Geometry check sheet. Reference: the model listing, model coordinates, mm. A direction names the side the tool comes from. Coordinates: 2 decimals unless noted, no trailing zeros. Write each loop counter-clockwise with the first axis right and the second up, starting at its lowest first coordinate (ties: lowest second). Pieces come first, ordered by that corner, then holes. Notation, with made-up numbers: M -38.5,34.5 L -14.5,34.5 A28 ccw -14.5,53.5 Z; hole C 76.25,80 d3. An arc over 180 degrees is marked long. Answer as a JSON object with one key per item and string values. Group by question number.
Autodesk Fusion 360 part; units mm, degrees
sketch "Sketch1" plane through (0, 0, 0) normal (0, 0, 1) x (1, 0, 0)
  line L0 (0, 0) -> (-70, 0)
  line L1 (-70, 0) -> (-70, 45)
  line L2 (-70, 45) -> (0, 45)
  line L3 (0, 45) -> (0, 0)
extrude "Extrude1" add sketch "Sketch1" along normal blind 75
sketch "Sketch2" plane through (0, 0, 75) normal (0, 0, 1) x (-1, 0, 0)
  line L0 (0, -45) -> (70, -45)
  line L1 (70, -45) -> (70, 0)
  line L2 (70, 0) -> (0, 0)
  line L3 (0, 0) -> (0, -45)
  line L4 (68, -43) -> (2, -43)
  line L5 (2, -43) -> (2, -2)
  line L6 (2, -2) -> (68, -2)
  line L7 (68, -2) -> (68, -43)
extrude "Extrude2" cut sketch "Sketch2" against normal blind 74.8 contours L4 L5 L6 L7
sketch "Sketch3" plane through (0, 0, 0.2) normal (0, 0, 1) x (-1, 0, 0)
  line L0 (68, -2) -> (2, -2)
  line L1 (2, -2) -> (2, -43)
  line L2 (2, -43) -> (68, -43)
  line L3 (68, -43) -> (68, -2)
  line L4 (68, -21) -> (65, -21)
  line L5 (65, -21) -> (65, -20)
  line L6 (65, -20) -> (68, -20)
  line L7 (68, -20) -> (68, -21)
  line L8 (67, -21) -> (68, -21)
  line L9 (68, -21) -> (68, -22)
  line L10 (68, -22) -> (67, -22)
  line L11 (67, -22) -> (67, -21)
  line L12 (68, -23) -> (65, -23)
  line L13 (65, -23) -> (65, -22)
  line L14 (65, -22) -> (68, -22)
  line L15 (68, -22) -> (68, -23)
  line L16 (19, -22) -> (16, -22)
  line L17 (16, -22) -> (16, -23)
  line L18 (16, -23) -> (19, -23)
  line L19 (19, -23) -> (19, -22)
  line L20 (17, -22) -> (16, -22)
  line L21 (16, -22) -> (16, -21)
  line L22 (16, -21) -> (17, -21)
  line L23 (17, -21) -> (17, -22)
  line L24 (16, -21) -> (19, -21)
  line L25 (19, -21) -> (19, -20)
  line L26 (19, -20) -> (16, -20)
  line L27 (16, -20) -> (16, -21)
extrude "Extrude3" add sketch "Sketch3" along normal blind 74 contours L3 L4 L5 L6 L7 L8 | L3 L4 L8 L9 L10 L11 L14 | L3 L10 L12 L13 L14 L15 | L16 L17 L18 L19 L20 | L16 L20 L21 L22 L23 L24 | L22 L24 L25 L26 L27
sketch "Sketch4" plane through (-68, 0, 0) normal (1, 0, 0) x (0, 1, 0)
  line L0 (23, 74.2) -> (23, 0.2)
  line L1 (23, 0.2) -> (43, 0.2)
  line L2 (43, 0.2) -> (43, 75)
  line L3 (43, 75) -> (2, 75)
  line L4 (2, 75) -> (2, 0.2)
  line L5 (2, 0.2) -> (20, 0.2)
  line L6 (20, 0.2) -> (20, 74.2)
  line L7 (20, 74.2) -> (23, 74.2)
  line L8 (28, 72) -> (42, 72)
  line L9 (42, 72) -> (42, 62)
  line L10 (42, 62) -> (28, 62)
  line L11 (28, 62) -> (28, 72)
extrude "Extrude4" cut sketch "Sketch4" against normal blind 8 contours L8 L9 L10 L11
sketch "Sketch5" plane through (0, 0, 0) normal (1, 0, 0) x (0, 1, 0)
  line L0 (0, 0) -> (45, 0)
  line L1 (45, 0) -> (45, 75)
  line L2 (45, 75) -> (0, 75)
  line L3 (0, 75) -> (0, 0)
  line L4 (42, 72) -> (28, 72)
  line L5 (28, 72) -> (28, 62)
  line L6 (28, 62) -> (42, 62)
  line L7 (42, 62) -> (42, 72)
extrude "Extrude5" cut sketch "Sketch5" against normal blind 9 contours L4 L5 L6 L7
sketch "Sketch6" plane through (0, 43, 0) normal (0, -1, 0) x (1, 0, 0)
  line L0 (-2, 75) -> (-68, 75)
  line L1 (-68, 75) -> (-68, 0.2)
  line L2 (-68, 0.2) -> (-2, 0.2)
  line L3 (-2, 0.2) -> (-2, 75)
  line L4 (-41, 75) -> (-25, 75)
  line L5 (-25, 75) -> (-25, 66)
  line L6 (-25, 66) -> (-41, 66)
  line L7 (-41, 66) -> (-41, 75)
extrude "Extrude6" cut sketch "Sketch6" against normal blind 8 contours L0 L4 L5 L6 L7
sketch "Sketch7" plane through (0, 0, 0) normal (0, 0, -1) x (1, 0, 0)
  line L0 (-70, -45) -> (0, -45)
  line L1 (0, -45) -> (0, 0)
  line L2 (0, 0) -> (-70, 0)
  line L3 (-70, 0) -> (-70, -45)
  line L4 (-64, -5) -> (-60, -5)
  line L5 (-60, -5) -> (-60, -7)
  line L6 (-60, -7) -> (-64, -7)
  line L7 (-64, -7) -> (-64, -5)
  line L8 (-64, -40) -> (-60, -40)
  line L9 (-60, -40) -> (-60, -38)
  line L10 (-60, -38) -> (-64, -38)
  line L11 (-64, -38) -> (-64, -40)
  line L12 (-6, -5) -> (-10, -5)
  line L13 (-10, -5) -> (-10, -7)
  line L14 (-10, -7) -> (-6, -7)
  line L15 (-6, -7) -> (-6, -5)
  line L16 (-6, -38) -> (-10, -38)
  line L17 (-10, -38) -> (-10, -40)
  line L18 (-10, -40) -> (-6, -40)
  line L19 (-6, -40) -> (-6, -38)
extrude "Extrude7" add sketch "Sketch7" along normal blind 4 contours L4 L5 L6 L7 | L8 L9 L10 L11 | L12 L13 L14 L15 | L16 L17 L18 L19
sketch "Sketch8" plane through (0, 7, 0) normal (0, 1, 0) x (-1, 0, 0)
  line L0 (64, 0) -> (60, 0)
  line L1 (60, 0) -> (60, -4)
  line L2 (60, -4) -> (64, -4)
  line L3 (64, -4) -> (64, 0)
  line L4 (64, -4) -> (60, -4)
  line L5 (60, -4) -> (60, -2)
  line L6 (60, -2) -> (64, -2)
  line L7 (64, -2) -> (64, -4)
extrude "Extrude8" add sketch "Sketch8" along normal blind 31 contours L1 L2 L3 L4 L5 L6 L7
sketch "Sketch9" plane through (0, 7, 0) normal (0, 1, 0) x (-1, 0, 0)
  line L0 (10, 0) -> (6, 0)
  line L1 (6, 0) -> (6, -4)
  line L2 (6, -4) -> (10, -4)
  line L3 (10, -4) -> (10, 0)
  line L4 (10, -4) -> (6, -4)
  line L5 (6, -4) -> (6, -2)
  line L6 (6, -2) -> (10, -2)
  line L7 (10, -2) -> (10, -4)
extrude "Extrude9" add sketch "Sketch9" along normal blind 31 contours L1 L2 L3 L4 L5 L6 L7
sketch "Sketch10" plane through (0, 0, 0.2) normal (0, 0, 1) x (-1, 0, 0)
  line L0 (68, -23) -> (65, -23)
  line L1 (65, -23) -> (65, -22)
  line L2 (65, -22) -> (67, -22)
  line L3 (67, -22) -> (67, -21)
  line L4 (67, -21) -> (65, -21)
  line L5 (65, -21) -> (65, -20)
  line L6 (65, -20) -> (68, -20)
  line L7 (68, -20) -> (68, -2)
  line L8 (68, -2) -> (2, -2)
  line L9 (2, -2) -> (2, -43)
  line L10 (2, -43) -> (68, -43)
  line L11 (68, -43) -> (68, -23)
  line L12 (17, -21) -> (17, -22)
  line L13 (17, -22) -> (19, -22)
  line L14 (19, -22) -> (19, -23)
  line L15 (19, -23) -> (16, -23)
  line L16 (16, -23) -> (16, -20)
  line L17 (16, -20) -> (19, -20)
  line L18 (19, -20) -> (19, -21)
  line L19 (19, -21) -> (17, -21)
  line L20 (2, -21) -> (3, -21)
  line L21 (3, -21) -> (3, -24)
  line L22 (3, -24) -> (2, -24)
  line L23 (2, -24) -> (2, -21)
  line L24 (3, -24) -> (5, -24)
  line L25 (5, -24) -> (5, -23)
  line L26 (5, -23) -> (3, -23)
  line L27 (3, -23) -> (3, -24)
  line L28 (3, -21) -> (5, -21)
  line L29 (5, -21) -> (5, -22)
  line L30 (5, -22) -> (3, -22)
  line L31 (3, -22) -> (3, -21)
  line L32 (45, -43) -> (46, -43)
  line L33 (46, -43) -> (46, -40)
  line L34 (46, -40) -> (45, -40)
  line L35 (45, -40) -> (45, -43)
  line L36 (46, -43) -> (47, -43)
  line L37 (47, -43) -> (47, -42)
  line L38 (47, -42) -> (46, -42)
  line L39 (46, -42) -> (46, -43)
  line L40 (48, -43) -> (47, -43)
  line L41 (47, -43) -> (47, -40)
  line L42 (47, -40) -> (48, -40)
  line L43 (48, -40) -> (48, -43)
  line L44 (45, -2) -> (46, -2)
  line L45 (46, -2) -> (46, -5)
  line L46 (46, -5) -> (45, -5)
  line L47 (45, -5) -> (45, -2)
  line L48 (46, -2) -> (47, -2)
  line L49 (47, -2) -> (47, -3)
  line L50 (47, -3) -> (46, -3)
  line L51 (46, -3) -> (46, -2)
  line L52 (47, -2) -> (48, -2)
  line L53 (48, -2) -> (48, -5)
  line L54 (48, -5) -> (47, -5)
  line L55 (47, -5) -> (47, -2)
extrude "Extrude10" add sketch "Sketch10" along normal blind 74 contours L10 L37 L40 L41 L42 L43 | L10 L33 L36 L37 L38 L39 L41 | L10 L32 L33 L34 L35 L39 | L9 L20 L21 L22 L23 L27 L31 | L21 L24 L25 L26 L27 | L8 L49 L52 L53 L54 L55 | L21 L28 L29 L30 L31 | L8 L45 L48 L49 L50 L51 L55 | L8 L44 L45 L46 L47 L51
sketch "Sketch11" plane through (0, 45, 0) normal (0, 1, 0) x (-1, 0, 0)
  line L0 (25, 66) -> (25, 75)
  line L1 (41, 75) -> (41, 66)
  line L2 (41, 66) -> (25, 66)
  line L3 (0, 0) -> (70, 0)
  line L4 (70, 0) -> (70, 75)
  line L5 (25, 75) -> (0, 75)
  line L6 (0, 75) -> (0, 0)
  line L7 (25, 66) -> (21, 66)
  line L8 (21, 66) -> (21, 72)
  line L9 (21, 72) -> (25, 72)
  line L10 (25, 72) -> (25, 66)
  line L11 (70, 75) -> (41, 75)
extrude "Extrude11" cut sketch "Sketch11" against normal blind 4 contours L0 L7 L8 L9 L10
extrude "Extrude12" add sketch "Sketch11" against normal blind 2 contours L0 L7 L8 L9 L10
1) Section check C-C (z = 5). State how many separate pieces and enclosed holes the cut face has, then the cut area to 3 significant figures.
2) Section check D-D (y = 34.5). Record the cut outline in (x, z), then the cut area to 3 significant figures.
3) Go/stop test with flat-tipped pins: pin 1 Ø13.5 at (x, y) = (-22.5, 32) entering from -Z; pin 2 Ø2 at (x, y) = (-43.5, 23.5) entering from +Z; pin 3 Ø1 at (x, z) = (-9, -1) entering from -Y. Record where each tip stops, or that it passes through.
4) Section check B-B (x = -23.5). Record the cut outline in (y, z), then the cut area to 3 significant figures.
5) Draft check along Z on faces 1 (the flat face through (-3, 21, 37)), 2 (the flat face through (-69, 35, 72)), 3 (the flat face through (-33, 44, 66)). Enter one of: +Z half, -Z half, draft (parallel to the pull), parting line (faces both ways), or undercut.
6) Material ranges on probe 1 along X at (y, z) = (42.5, 25); probe 2 along Y at (x, z) = (-24, 45); probe 3 along X at (y, z) = (13, 35), recorded low to high. Write a range as [from, to].
7) Section check A-A (y = 8). Record the cut outline in (x, z).
8) Set-up check for faces 4 (the flat face through (-62, 5, -2)), 5 (the flat face through (-64, 22, -3)), 6 (the flat face through (-41, 44, 70)), 7 (the flat face through (-8, 40, -2)), 8 (the flat face through (-46.5, 2.8, 74.2)): record each of +Z, -Z, +X, -X, +Y, -Y from which the full face is reachable in a straight line by a thin tool's end or side.
Entries:
{
 "1": {"separate pieces": "2", "enclosed holes": "1", "area": "479 mm^2"},
 "2": {"outline": "M -70,0 L 0,0 L 0,62 L -2,62 L -2,0.2 L -68,0.2 L -68,62 L -70,62 Z; M -70,72 L -68,72 L -68,75 L -70,75 Z; M -64,-4 L -60,-4 L -60,-2 L -64,-2 Z; M -10,-4 L -6,-4 L -6,-2 L -10,-2 Z; M -2,72 L 0,72 L 0,75 L -2,75 Z", "area": "289 mm^2"},
 "3": {"pin 1": "z = 0", "pin 2": "z = 0.2", "pin 3": "y = 5"},
 "4": {"outline": "M 0,0 L 45,0 L 45,75 L 43,75 L 43,0.2 L 2,0.2 L 2,75 L 0,75 Z", "area": "308 mm^2"},
 "5": {"face 1": "draft", "face 2": "undercut", "face 3": "+Z half"},
 "6": {"probe 1": "[-70, -68], [-48, -45], [-2, 0]", "probe 2": "[0, 2], [43, 45]", "probe 3": "[-70, -68], [-2, 0]"},
 "7": {"outline": "M -70,0 L 0,0 L 0,75 L -2,75 L -2,0.2 L -68,0.2 L -68,75 L -70,75 Z; M -64,-4 L -60,-4 L -60,-2 L -64,-2 Z; M -10,-4 L -6,-4 L -6,-2 L -10,-2 Z"},
 "8": {"face 4": "-Z, +X, -X, -Y", "face 5": "-Z, -X, +Y, -Y", "face 6": "+Z, +Y", "face 7": "-Z, +X, -X, +Y", "face 8": "+Z"}
}
